Here's how the part is built. I have some questions about the finished solid (model axes, mm). Face numbers are marked on the shaded views. A direction names the side the tool comes from. Round coordinates to 2 decimals unless told otherwise and drop trailing zeros. Loops run counter-clockwise (first coordinate to the right, second up) from the corner with the lowest first, then second, coordinate; pieces in that order, holes last. Notation, with made-up numbers: (38.25, 55) -> (63.25, 55) arc R12 cw to (63.25, 66) -> close; hole circle Ø1 at (-34.5, 11). An arc over 180 degrees is marked (long way). Use one line per item in the form item = value. Start each with the question number.
Item 1: If we section it at A-A (y = -50): Write out the boundary of the cut face in (x, z), then the cut area to 3 significant figures.
Item 2: Thinking about a two-plate mould opening in Z: for the marked faces 1, 2 and 3, which applies, released by +Z, released by -Z, zero draft, split by the parting line, or undercut?
Item 3: For the marked faces 4 and 5, which set-ups out of +Z, -Z, +X, -X, +Y, -Y let a thin tool reach every point of the face, with its end or its side?
Item 4: If I drill on L1, parallel to Y at x = 0, z = 6; L2, parallel to Y at x = 1.25, z = 8; L3, parallel to Z at x = -0.5, y = -50, over which ranges is the centre line in solid material (lowest first)? Write a range as [from, to].
Item 5: I'm going to push flat-ended pins straight in: pin 1 Ø6 at (x, z) = (-1, 18.5) entering from -Y; pin 2 Ø5 at (x, y) = (-3.5, -7.5) entering from +Z; pin 3 Ø2 at (x, y) = (3.5, -22.5) entering from -Z; pin 4 Ø1.2 at (y, z) = (-62, 19.5) entering from +X. Where does each tip first touch, or does it pass through?
Item 6: If we section it at D-D (x = -1.25): Write out the boundary of the cut face in (y, z).
Item 7: If we section it at B-B (x = -6): Write out the boundary of the cut face in (y, z), then the cut area to 3 significant figures.
Item 8: If we section it at C-C (z = 8): Write out the boundary of the cut face in (x, y).
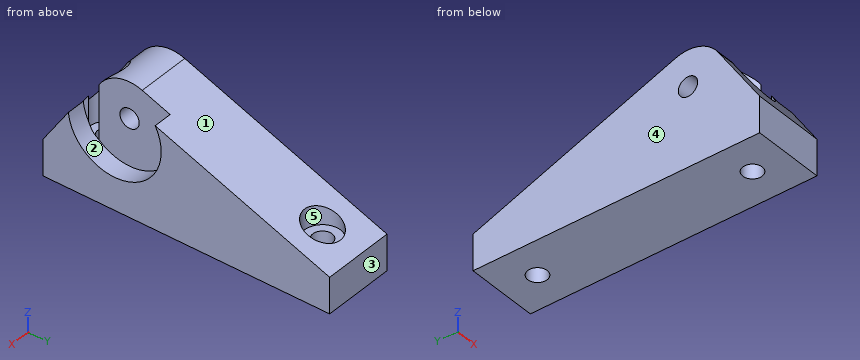
```python
from build123d import *

# Parameters (mm, degrees)
SKETCH1_W           = 20
SKETCH1_H           = 80
SKETCH1_R           = 2.7
BOSS_EXTRUDE1_DEPTH = 10
SKETCH2_R           = 2.7
BOSS_EXTRUDE2_DEPTH = 10
SKETCH3_R           = 5
CUT_EXTRUDE1_DEPTH  = 23
SKETCH4_R           = 13
CUT_EXTRUDE2_DEPTH  = 5.2


with BuildPart() as part:
    # Sketch1 → Boss-Extrude1 (new body)
    with BuildSketch(Plane.XY):
        with Locations((0, -30)):
            Rectangle(SKETCH1_W, SKETCH1_H)
        Circle(SKETCH1_R, mode=Mode.SUBTRACT)
        with Locations((0, -60)):
            Circle(SKETCH1_R, mode=Mode.SUBTRACT)
    extrude(amount=BOSS_EXTRUDE1_DEPTH)

    # Sketch2 → Boss-Extrude2 (add, symmetric)
    with BuildSketch(Plane(origin=(0, 0, 0), x_dir=(0, 0, -1), z_dir=(1, 0, 0))):
        with BuildLine():
            Line((-10, 10), (-31.353454021, -46.462642529))
            ThreePointArc((-31.353454021, -46.462642529), (-31.520338182, -53.05992825), (-27.540921877, -58.324553126))
            Line((-27.540921877, -58.324553126), (-10, -70))
            Line((-10, -70), (-10, 10))
        make_face()
        with Locations((-22, -50)):
            Circle(SKETCH2_R, mode=Mode.SUBTRACT)
    extrude(amount=BOSS_EXTRUDE2_DEPTH, both=True)

    # Sketch3 → Cut-Extrude1 (cut, through all)
    with BuildSketch(Plane(origin=(0, 0, 10), x_dir=(-1, 0, 0), z_dir=(0, 0, -1))):
        with Locations((0, -60)):
            Circle(SKETCH3_R)
        Circle(SKETCH3_R)
    extrude(amount=-CUT_EXTRUDE1_DEPTH, mode=Mode.SUBTRACT)

    # Sketch4 → Cut-Extrude2 (cut)
    with BuildSketch(Plane(origin=(10, 0, 0), x_dir=(0, 0, -1), z_dir=(1, 0, 0))):
        with Locations((-22, -50)):
            Circle(SKETCH4_R)
    extrude(amount=-CUT_EXTRUDE2_DEPTH, mode=Mode.SUBTRACT)


solid = part.part
```
Values found:
q1.outline = (-10, 0) -> (10, 0) -> (10, 9) -> (4.8, 9) -> (4.8, 19.3) -> (-10, 19.3) -> close; (-10, 24.7) -> (4.8, 24.7) -> (4.8, 32) -> (-10, 32) -> close
q1.area = 440 mm2
q2.face_1 = released by +Z
q2.face_2 = undercut
q2.face_3 = zero draft
q3.face_4 = +Z, -Z, -X, +Y, -Y
q3.face_5 = +Z
q4.L1 = [-70, -62.7], [-57.3, -2.7], [2.7, 10]
q4.L2 = [-70, -62.39], [-57.61, -2.39], [2.39, 10]
q4.L3 = [0, 19.3], [24.7, 32]
q5.pin_1 = -66.34
q5.pin_2 = 17.56
q5.pin_3 = 0
q5.pin_4 = 4.8
q6.outline = (-70, 0) -> (-62.39, 0) -> (-62.39, 10) -> (-64.84, 10) -> (-64.84, 17.75) -> (-70, 10) -> close; (-57.61, 0) -> (-2.39, 0) -> (-2.39, 10) -> (-4.84, 10) -> (-4.84, 15.61) -> (-46.46, 31.35) arc R10 ccw to (-55.16, 30.57) -> (-55.16, 10) -> (-57.61, 10) -> close; (2.39, 0) -> (10, 0) -> (10, 10) -> (4.84, 11.95) -> (4.84, 10) -> (2.39, 10) -> close; hole circle Ø5.4 at (-50, 22)
q7.outline = (-70, 0) -> (10, 0) -> (10, 10) -> (-46.46, 31.35) arc R10 ccw to (-58.32, 27.54) -> (-70, 10) -> close; hole circle Ø5.4 at (-50, 22)
q7.area = 1,730 mm2
q8.outline = (-10, -70) -> (10, -70) -> (10, 10) -> (-10, 10) -> close; hole circle Ø5.4 at (0, -60); hole circle Ø5.4 at (0, 0)
